Can you work these out from the drawing? Everything is in mm from the part's minimum corner. Round coordinates to 2 decimals unless told otherwise and drop trailing zeros. Order: outer loops, then holes, each group sorted by start corner. A loop starts at its lowest first (then second) coordinate and runs counter-clockwise, first axis right, second up. Notation, with made-up numbers: (25.25, 64) -> (62.25, 64) arc R26 ccw to (62.25, 87) -> close; hole circle Ø6 at (-12, -30.5). An arc over 180 degrees is marked (long way). One line per item, written item: value.
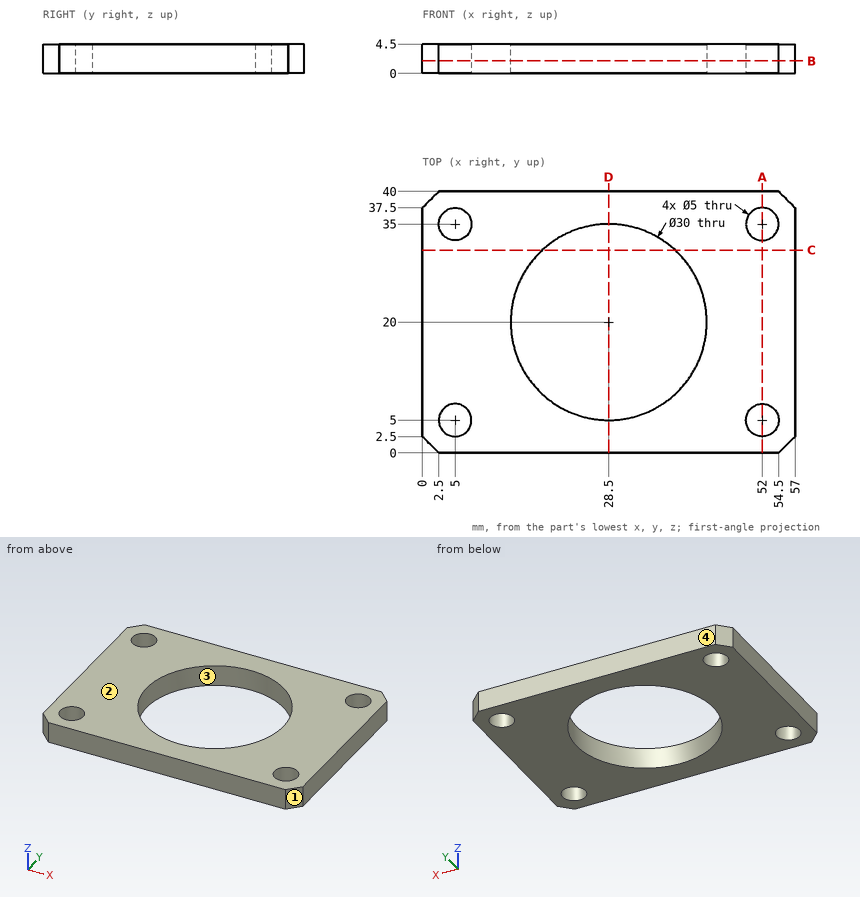
Q1. I need wall thicknesses on line 1 along Y through (x, z) = (5, 3.4); line 2 along X through (y, z) = (36, 2.4); line 3 along X through (y, z) = (7, 3.6). Which ranges of each line are inside material? Lowest first, please.
Answers:
line 1: 0 to 2.5, 7.5 to 32.5, 37.5 to 40
line 2: 0 to 2.71, 7.29 to 49.71, 54.29 to 57
line 3: 0 to 3.5, 6.5 to 21.02, 35.98 to 50.5, 53.5 to 57
Q2. I want a section at A-A on x = 52. Write out the boundary of the cut face in (y, z), then the cut area to 3 significant figures.
Answers:
outline: (0, 0) -> (2.5, 0) -> (2.5, 4.5) -> (0, 4.5) -> close; (7.5, 0) -> (32.5, 0) -> (32.5, 4.5) -> (7.5, 4.5) -> close; (37.5, 0) -> (40, 0) -> (40, 4.5) -> (37.5, 4.5) -> close
area: 135 mm2
Q3. If we mould it in two halves opening along Y, with no side actions, what happens to the marked faces 1, 2, 3 and 4? For each: pulls with the +Y half, pulls with the -Y half, needs draft (parallel to the pull), parting line crosses it, or undercut.
Answers:
face 1: pulls with the -Y half
face 2: needs draft
face 3: undercut
face 4: pulls with the +Y half
Q4. I want a section at C-C on y = 31. Write out the boundary of the cut face in (x, z).
Answers:
outline: (0, 0) -> (18.3, 0) -> (18.3, 4.5) -> (0, 4.5) -> close; (38.7, 0) -> (57, 0) -> (57, 4.5) -> (38.7, 4.5) -> close
Q5. I want a section at B-B on z = 1.9. Write out the boundary of the cut face in (x, y), then the cut area to 3 significant figures.
Answers:
outline: (0, 2.5) -> (2.5, 0) -> (54.5, 0) -> (57, 2.5) -> (57, 37.5) -> (54.5, 40) -> (2.5, 40) -> (0, 37.5) -> close; hole circle Ø5 at (5, 5); hole circle Ø5 at (5, 35); hole circle Ø30 at (28.5, 20); hole circle Ø5 at (52, 5); hole circle Ø5 at (52, 35)
area: 1,480 mm2
Q6. I want a section at D-D on x = 28.5. Write out the boundary of the cut face in (y, z).
Answers:
outline: (0, 0) -> (5, 0) -> (5, 4.5) -> (0, 4.5) -> close; (35, 0) -> (40, 0) -> (40, 4.5) -> (35, 4.5) -> close
Q7. For P1, Ø6, axis at x = 52, y = 5, coming from the -Z side; P2, Ø3, axis at x = 5, y = 35, coming from the -Z side, each with a flat end and sliding along its axis, tell me the tip position at first contact or that it passes through.
Answers:
P1: z = 0
P2: through
